Work out the finished part from the listing and answer in its coordinate system (mm). A direction names the side the tool comes from. Give positions to 0.01 mm unless a question says otherwise; leave off trailing zeros. Order: outer loops, then holes, each group sorted by start corner. A loop starts at its lowest first (then second) coordinate and runs counter-clockwise, first axis right, second up.
```python
from build123d import *

# Parameters (mm, degrees)
SKETCH1_W           = 54
SKETCH1_H           = 25
SKETCH1_W_2         = 52
SKETCH1_H_2         = 23
BOSS_EXTRUDE1_DEPTH = 5
SKETCH2_W           = 54
SKETCH2_H           = 25
SKETCH2_R           = 1.4
BOSS_EXTRUDE2_DEPTH = 2.2
SKETCH3_W           = 44.75
SKETCH3_H           = 23.07193706
CUT_EXTRUDE1_DEPTH  = 1.7
FILLET1_R           = 1
SKETCH5_W           = 2
SKETCH5_H           = 23.07193706
BOSS_EXTRUDE3_DEPTH = 3.2


with BuildPart() as part:
    # Sketch1 → Boss-Extrude1 (new body)
    with BuildSketch(Plane.XY):
        Rectangle(SKETCH1_W, SKETCH1_H)
        Rectangle(SKETCH1_W_2, SKETCH1_H_2, mode=Mode.SUBTRACT)
    extrude(amount=BOSS_EXTRUDE1_DEPTH)

    # Sketch2 → Boss-Extrude2 (add)
    with BuildSketch(Plane(origin=(0, 0, 0), x_dir=(-1, 0, 0), z_dir=(0, 0, -1))):
        Rectangle(SKETCH2_W, SKETCH2_H)
        with Locations((24, 8.25)):
            Circle(SKETCH2_R, mode=Mode.SUBTRACT)
        with Locations((24, -8.25)):
            Circle(SKETCH2_R, mode=Mode.SUBTRACT)
        with Locations((-23, 8.25)):
            Circle(SKETCH2_R, mode=Mode.SUBTRACT)
        with Locations((-23, -8.25)):
            Circle(SKETCH2_R, mode=Mode.SUBTRACT)
        with BuildLine():
            Line((-11.25, -9.75), (18.75, -9.75))
            ThreePointArc((18.75, -9.75), (20.871320344, -8.871320344), (21.75, -6.75))
            Line((21.75, -6.75), (21.75, 6.75))
            ThreePointArc((21.75, 6.75), (20.871320344, 8.871320344), (18.75, 9.75))
            Line((18.75, 9.75), (-11.25, 9.75))
            ThreePointArc((-11.25, 9.75), (-13.371320344, 8.871320344), (-14.25, 6.75))
            Line((-14.25, 6.75), (-14.25, -6.75))
            ThreePointArc((-14.25, -6.75), (-13.371320344, -8.871320344), (-11.25, -9.75))
        make_face(mode=Mode.SUBTRACT)
    extrude(amount=-BOSS_EXTRUDE2_DEPTH)

    # Sketch3 → Cut-Extrude1 (cut)
    with BuildSketch(Plane.XY.offset(2.2)):
        with Locations((3.625, -0.03596853)):
            Rectangle(SKETCH3_W, SKETCH3_H)
    extrude(amount=-CUT_EXTRUDE1_DEPTH, mode=Mode.SUBTRACT)

    # Fillet1
    fillet1_edges = [part.edges().sort_by_distance(p)[0] for p in [
        (-18.75, 10.625, 2.2),
    ]]
    fillet(fillet1_edges, radius=FILLET1_R)

    # Sketch5 → Boss-Extrude3 (add)
    with BuildSketch(Plane.XY.offset(0.5)):
        with Locations((19.5, -0.03596853)):
            Rectangle(SKETCH5_W, SKETCH5_H)
    extrude(amount=BOSS_EXTRUDE3_DEPTH)


solid = part.part
```
1. The part is cut by section C-C (x = -8.5). Write down the section's boundary in (y, z).
Findings below:
outline: (-12.5, 0) - (-9.75, 0) - (-9.75, 0.5) - (-11.57, 0.5) - (-11.57, 2.2) - (-11.5, 2.2) - (-11.5, 5) - (-12.5, 5) - close; (9.75, 0) - (12.5, 0) - (12.5, 5) - (11.5, 5) - (11.5, 0.5) - (9.75, 0.5) - close
2. The part is cut by section B-B (x = 23). Write down the section's boundary in (y, z).
Findings below:
outline: (-12.5, 0) - (-9.65, 0) - (-9.65, 0.5) - (-11.57, 0.5) - (-11.57, 2.2) - (-11.5, 2.2) - (-11.5, 5) - (-12.5, 5) - close; (-6.85, 0) - (6.85, 0) - (6.85, 0.5) - (-6.85, 0.5) - close; (9.65, 0) - (12.5, 0) - (12.5, 5) - (11.5, 5) - (11.5, 0.5) - (9.65, 0.5) - close
3. The part is cut by section A-A (y = -5.75). Write down the section's boundary in (x, z), then the cut area to 3 significant figures.
Findings below:
outline: (-27, 0) - (-21.75, 0) - (-21.75, 2.2) - (-26, 2.2) - (-26, 5) - (-27, 5) - close; (14.25, 0) - (27, 0) - (27, 5) - (26, 5) - (26, 0.5) - (20.5, 0.5) - (20.5, 3.7) - (18.5, 3.7) - (18.5, 0.5) - (14.25, 0.5) - close
area: 31.6 mm2
4. Straight lines are drawn through the part: probe 1 along X at (y, z) = (-0.25, 2); probe 2 along X at (y, z) = (10.75, 1.1); probe 3 along Y at (x, z) = (23, 0.3). For each, find the intervals that lie inside material, in ascending order.
Findings below:
probe 1: x = -27 to -21.75, 18.5 to 20.5, 26 to 27
probe 2: x = -27 to -18.75, 18.5 to 20.5, 26 to 27
probe 3: y = -12.5 to -9.65, -6.85 to 6.85, 9.65 to 12.5
5. The mould has two halves that part along Z. Classify faces 4 (the face through (27, 0, 2)), 5 (the face through (19, 0, 3.7)), 6 (the face through (0, -11.572, 1)): pulls with the +Z half, pulls with the -Z half, needs draft (parallel to the pull), parting line crosses it, or undercut.
Findings below:
face 4: needs draft
face 5: pulls with the +Z half
face 6: undercut
6. Which of the six approach directions +Z, -Z, +X, -X, +Y, -Y give full straight-line access (tool end or side, diameter ignored) to faces 1 (the face through (-21.75, 0, 1)), 2 (the face through (0, 11.5, 3)), 3 (the face through (23, -11.572, 1))?
Findings below:
face 1: +Z, -Z
face 2: +Z
face 3: none
7. Given P1, Ø6, axis at x = 22.5, y = -1, coming from the +Z side; P2, Ø1.5, axis at x = 10, y = -8.5, coming from the +Z side, each flat-ended and moving along its own axis, determine where each tip first touches the part or whether it passes through.
Findings below:
P1: stops at z = 3.7
P2: passes through
8. The part is cut by section D-D (y = -8.25). Write down the section's boundary in (x, z).
Findings below:
outline: (-27, 0) - (-25.4, 0) - (-25.4, 2.2) - (-26, 2.2) - (-26, 5) - (-27, 5) - close; (-22.6, 0) - (-21.35, 0) - (-21.35, 2.2) - (-22.6, 2.2) - close; (13.85, 0) - (21.6, 0) - (21.6, 0.5) - (20.5, 0.5) - (20.5, 3.7) - (18.5, 3.7) - (18.5, 0.5) - (13.85, 0.5) - close; (24.4, 0) - (27, 0) - (27, 5) - (26, 5) - (26, 0.5) - (24.4, 0.5) - close
